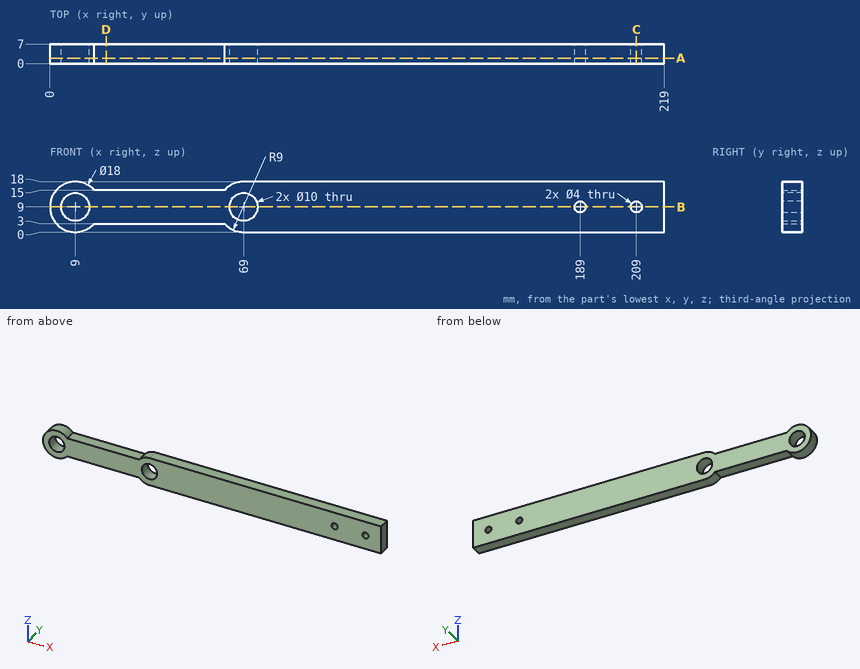
For this review, use the dimensioned drawing (mm, ordinates from the lowest corner) and the shaded views. Round coordinates to 2 decimals unless told otherwise and drop trailing zeros. Write each loop counter-clockwise with the first axis right and the second up, starting at its lowest first coordinate (ties: lowest second). Pieces come first, ordered by that corner, then holes. Notation, with made-up numbers: M -6,79.25 L 37,79.25 A23 cw 37,106.25 Z; hole C 34.25,82 d5. An arc over 180 degrees is marked long. Use CSV: the item, a comma, the result in double quotes. Start each with the question number.
(1) We need section B-B, the plane z = 9. State the section outline as (x, y) points, then the cut area to 3 significant figures.
(2) We need section D-D, the plane x = 20. State the section outline as (y, z) points.
(3) Clearance check with flat-ended pins moving along their axes: P1, Ø1.5, axis at y = 2.5, z = 5.5, coming from the -X side; P2, Ø2, axis at x = 43.5, y = 3.5, coming from the +Z side; P3, Ø3.5, axis at x = 48.5, y = 2, coming from the -Z side. State where each tip first meets the part, or that it passes through.
(4) We need section A-A, the plane y = 2. State the section outline as (x, z) points.
(5) For line 1 along X through (y, z) = (5, 9); line 2 along X through (y, z) = (0.75, 7.75); line 3 along Z through (x, y) = (209, 5), list the stretches that pass through material, from the lowest coordinate up.
(6) We need section C-C, the plane x = 209. State the section outline as (y, z) points, then the cut area to 3 significant figures.
Findings:
1,outline,"M 0,0 L 4,0 L 4,7 L 0,7 Z; M 14,0 L 64,0 L 64,7 L 14,7 Z; M 74,0 L 187,0 L 187,7 L 74,7 Z; M 191,0 L 207,0 L 207,7 L 191,7 Z; M 211,0 L 219,0 L 219,7 L 211,7 Z"
1,area,"1,340 mm^2"
2,outline,"M 0,3 L 7,3 L 7,15 L 0,15 Z"
3,P1,"x = 0.43"
3,P2,"z = 15"
3,P3,"z = 3"
4,outline,"M 15.71,3 L 62.29,3 A9 ccw 69,0 L 219,0 L 219,18 L 69,18 A9 ccw 62.29,15 L 15.71,15 A9 ccw long Z; hole C 9,9 d10; hole C 69,9 d10; hole C 189,9 d4; hole C 209,9 d4"
5,line 1,"0 to 4, 14 to 64, 74 to 187, 191 to 207, 211 to 219"
5,line 2,"0.09 to 4.16, 13.84 to 64.16, 73.84 to 187.44, 190.56 to 207.44, 210.56 to 219"
5,line 3,"0 to 7, 11 to 18"
6,outline,"M 0,0 L 7,0 L 7,7 L 0,7 Z; M 0,11 L 7,11 L 7,18 L 0,18 Z"
6,area,"98.0 mm^2"
